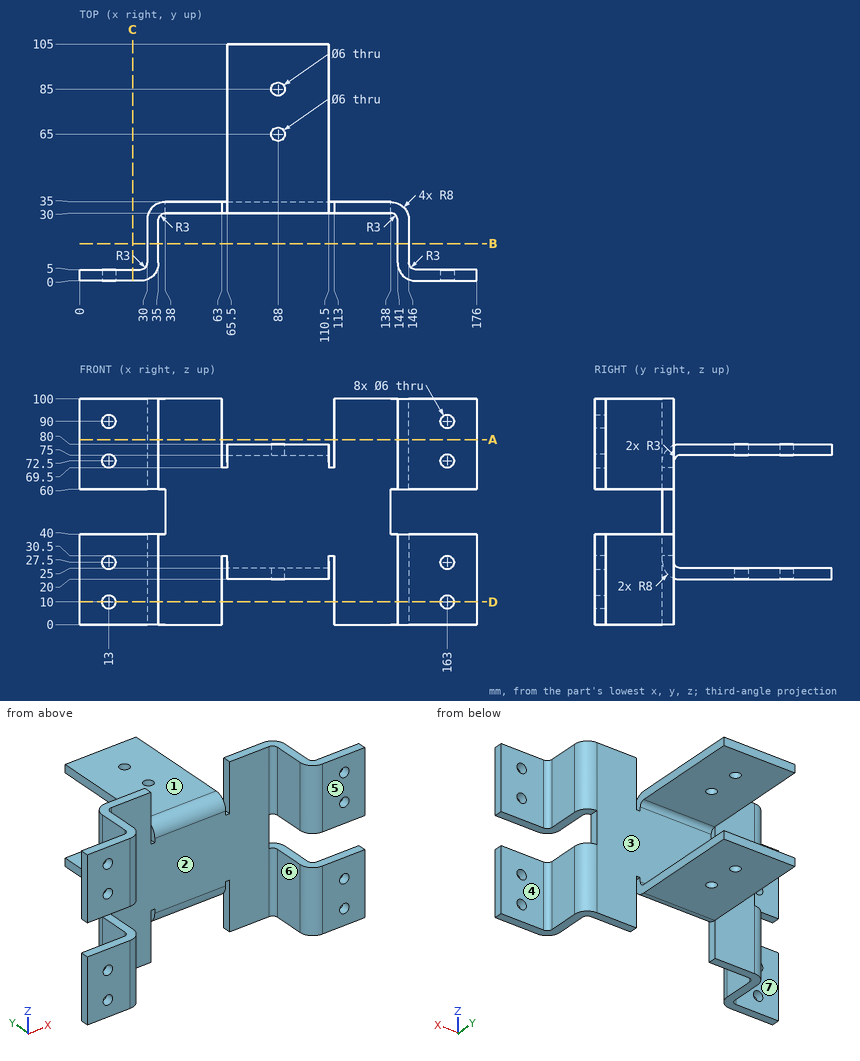
Answer from the drawing. Dimensions are ordinates in mm from the lowest x, y and z of the part. A direction names the side the tool comes from. Coordinates: 2 decimals unless noted, no trailing zeros. Write each loop counter-clockwise with the first axis right and the second up, starting at its lowest first coordinate (ties: lowest second). Pieces come first, ordered by that corner, then holes. Notation, with made-up numbers: M -14.75,87.25 L 14.25,87.25 A18 cw 14.25,116.25 Z; hole C -35.5,0.25 d6. An arc over 180 degrees is marked long. Use a Markdown table: item, result.
Q1. The part is cut by section A-A, the plane z = 82. Write down the section's boundary in (x, y), then the cut area to 3 significant figures.
Answer block:
| item | result |
|---|---|
| outline | M 0,0 L 27,0 A8 ccw 35,8 L 35,27 A3 cw 38,30 L 63,30 L 63,35 L 38,35 A8 ccw 30,27 L 30,8 A3 cw 27,5 L 0,5 Z; M 113,30 L 138,30 A3 cw 141,27 L 141,8 A8 ccw 149,0 L 176,0 L 176,5 L 149,5 A3 cw 146,8 L 146,27 A8 ccw 138,35 L 113,35 Z |
| area | 883 mm2 |
Q2. Determine the mould class of the marked faces 1, 2 and 3 for opening direction Z: released by +Z, released by -Z, zero draft, split by the parting line, or undercut.
Answer block:
| item | result |
|---|---|
| face 1 | released by +Z |
| face 2 | zero draft |
| face 3 | undercut |
Q3. The part is cut by section B-B, the plane y = 16.5. Write down the section's boundary in (x, z).
Answer block:
| item | result |
|---|---|
| outline | M 30,0 L 35,0 L 35,40 L 30,40 Z; M 30,60 L 35,60 L 35,100 L 30,100 Z; M 141,0 L 146,0 L 146,40 L 141,40 Z; M 141,60 L 146,60 L 146,100 L 141,100 Z |
Q4. Which of the six approach directions +Z, -Z, +X, -X, +Y, -Y give full straight-line access (tool end or side, diameter ignored) to the marked faces 4, 5, 6 and 7?
Answer block:
| item | result |
|---|---|
| face 4 | +Z, -Z, +X, +Y |
| face 5 | +Z, -Z, +X, -X, -Y |
| face 6 | +Z, -Z, -Y |
| face 7 | +Z, -Z, -X, +Y |
Q5. Straight lines are drawn through the part: L1, parallel to Z at x = 163, y = 3.55; L2, parallel to Z at x = 94, y = 54.5; L3, parallel to X at y = 85, z = 77.4. For each, find the intervals that lie inside material, in ascending order. Write a range as [from, to].
Answer block:
| item | result |
|---|---|
| L1 | z = [0, 7], [13, 24.5], [30.5, 40], [60, 69.5], [75.5, 87], [93, 100] |
| L2 | z = [20, 25], [75, 80] |
| L3 | x = [65.5, 85], [91, 110.5] |
Q6. Each of these flat-tipped pins is pushed along its axis until it touches: pin 1 Ø6 at (x, z) = (118, 39.5) entering from -Y; pin 2 Ø1.5 at (y, z) = (32, 18) entering from +X; pin 3 Ø10 at (x, y) = (66.5, 43.5) entering from +Z. Where does it stop, or does it pass through?
Answer block:
| item | result |
|---|---|
| pin 1 | stops at y = 30 |
| pin 2 | stops at x = 144.78 |
| pin 3 | stops at z = 80 |
Q7. The part is cut by section D-D, the plane z = 10. Give the number of separate pieces and of enclosed holes in the cut face, then the cut area to 3 significant figures.
Answer block:
| item | result |
|---|---|
| separate pieces | 4 |
| enclosed holes | 0 |
| area | 823 mm2 |
Q8. The part is cut by section C-C, the plane x = 23.5. Write down the section's boundary in (y, z).
Answer block:
| item | result |
|---|---|
| outline | M 0,0 L 5,0 L 5,40 L 0,40 Z; M 0,60 L 5,60 L 5,100 L 0,100 Z |
